Verification items for this drawing (mm, ordinates from the low corner). Give positions to 0.01 mm unless a question says otherwise; leave off trailing zeros. Loops run counter-clockwise (first coordinate to the right, second up) from the corner with the lowest first, then second, coordinate; pieces in that order, holes last. Notation, with made-up numbers: (11, 36) -> (46, 36) arc R23 ccw to (46, 66) -> close; hole circle Ø7 at (44, 60.25). An arc over 180 degrees is marked (long way). Answer as a JSON object with one key per item and string values.
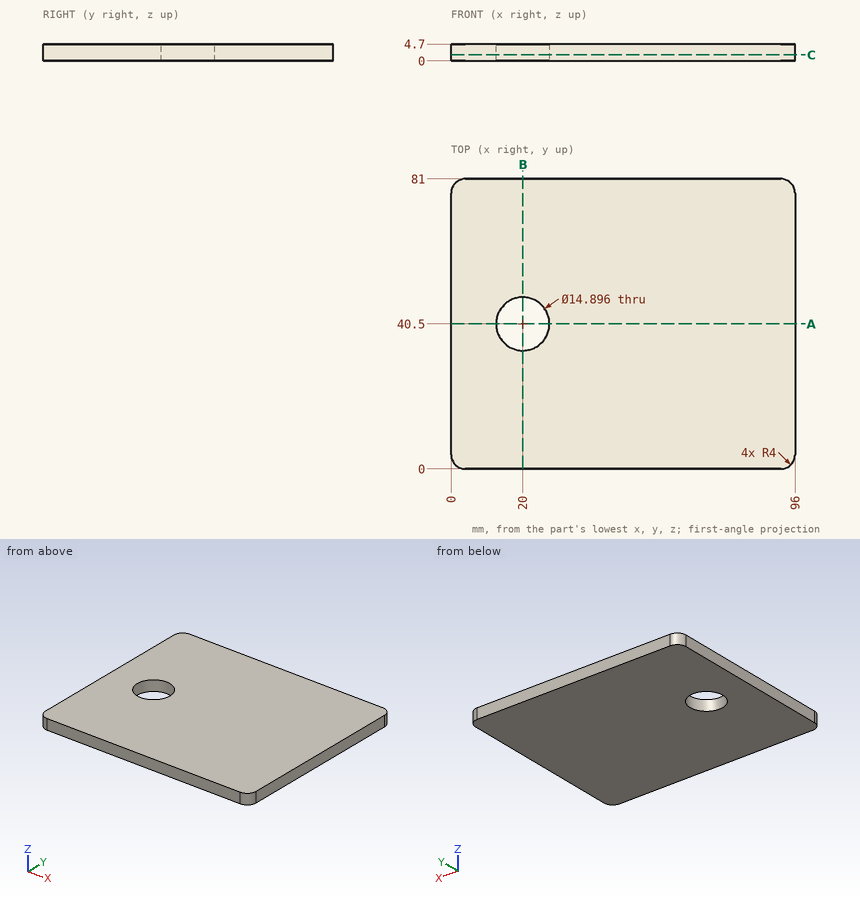
1) Section check C-C on z = 1.65. Record the cut outline in (x, y).
Geometry check:
{"outline": "(0, 4) arc R4 ccw to (4, 0) -> (92, 0) arc R4 ccw to (96, 4) -> (96, 77) arc R4 ccw to (92, 81) -> (4, 81) arc R4 ccw to (0, 77) -> close; hole circle Ø14.9 at (20, 40.5)"}
2) Section check A-A on y = 40.5. Record the cut outline in (x, z), plus the area to 3 significant figures.
Geometry check:
{"outline": "(0, 0) -> (12.55, 0) -> (12.55, 4.7) -> (0, 4.7) -> close; (27.45, 0) -> (96, 0) -> (96, 4.7) -> (27.45, 4.7) -> close", "area": "381 mm2"}
3) Material ranges on line 1 along Y through (x, z) = (20, 1.15); line 2 along X through (y, z) = (36, 0.4); line 3 along X through (y, z) = (78.5, 0.35), recorded low to high. Write a range as from..to.
Geometry check:
{"line 1": "y = 0..33.05, 47.95..81", "line 2": "x = 0..14.07, 25.93..96", "line 3": "x = 0.29..95.71"}
4) Section check B-B on x = 20. Record the cut outline in (y, z), plus the area to 3 significant figures.
Geometry check:
{"outline": "(0, 0) -> (33.05, 0) -> (33.05, 4.7) -> (0, 4.7) -> close; (47.95, 0) -> (81, 0) -> (81, 4.7) -> (47.95, 4.7) -> close", "area": "311 mm2"}
